Input: part model. Units: mm. Frame: model coordinates. A direction names the side the tool comes from. Coordinates: 2 decimals unless noted, no trailing zeros. Order: outer loops, then holes, each group sorted by start corner. A loop starts at its lowest first (then second) coordinate and runs counter-clockwise, first axis right, second up. Notation, with made-up numbers: (85.25, 70) -> (128.25, 70) arc R10 ccw to (128.25, 87) -> close; hole circle Ø4 at (25.5, 35). An arc over 180 degrees is marked (long way). Use one line per item in the form item = value. Start each with the question number.
1) Draft query along Y for faces 1 (the flat face through (-61.7, -38.656, 6.3)), 2 (the flat face through (-59.664, -5, 6)), 3 (the cylindrical face through (35.26, -34.87, 6.44)), 4 (the flat face through (-47, -1.432, 6)). Return one class per face: pulls with the +Y half, pulls with the -Y half, needs draft (parallel to the pull), parting line crosses it, or undercut.
2) Pin query (flat end, axial travel): pin 1 (3 mm diameter, centred on y = -6, z = 5, fed in from +X); pin 2 (7 mm diameter, centred on y = -5, z = 4, fed in from -X); pin 3 (4 mm diameter, centred on x = -7.5, z = 9, fed in from +Y). Return the tip coordinate at first contact, or that it passes through.
3) Section query A-A on y = -5.5. Output: boundary loops of the cut face in (x, z).
4) Section query D-D on x = -25.5. Output: boundary loops of the cut face in (y, z), then the cut area to 3 significant figures.
5) Section query B-B on z = 6.35. Count the separate pieces of the cut face and the enclosed holes in it, then the cut area to 3 significant figures.
6) Ray query, line 1 along Y through (x, z) = (-59, 1.5); line 2 along X through (y, z) = (-5.5, 6.35); line 3 along Z through (x, y) = (-52, -4). Return the intervals inside material, ascending.
7) Access query for faces 5 (the flat face through (47.2, -7.782, 7.7)), 6 (the flat face through (50.78, -5, 6)), 7 (the cylindrical face through (-48.168, -4.562, 5.129)). Directions: +Z, -Z, +X, -X, +Y, -Y. A direction counts if a zero-diameter tool reaches every point of the face in a straight line with its end or side. Return the directions, or none.
8) Section query C-C on x = 18. Output: boundary loops of the cut face in (y, z), then the cut area to 3 significant figures.
Autodesk Inventor part; units mm, degrees
ref_plane "YZ Plane" through (0, 0, 0) normal (1, 0, 0) x (0, 1, 0)
ref_plane "XZ Plane" through (0, 0, 0) normal (0, 1, 0) x (-1, 0, 0)
ref_plane "XY Plane" through (0, 0, 0) normal (0, 0, 1) x (1, 0, 0)
sketch "Sketch1" plane through (0, 0, 0) normal (0, 0, 1) x (1, 0, 0)
  arc A0 (-39.344, -1.4316) -> (30.4598, -1.4316) centre (-4.4421, -0.1616) ccw
  line L0 (-39.344, -1.4316) -> (-39.3671, -1.4316)
  line L1 (-39.344, -1.4316) -> (-52.044, -1.4316)
  line L2 (30.4598, -1.4316) -> (43.1598, -1.4316)
  arc A1 (-46.964, -22.4724) -> (38.0798, -22.4724) centre (-4.4421, -0.1616) ccw
  line L3 (-4.4421, -48.1813) -> (-4.4421, -51.3563)
  line L4 (-4.4421, -51.3563) -> (-72.364, -51.3563)
  line L5 (-4.4421, -51.3563) -> (63.4798, -51.3563)
  line L6 (-52.044, -1.4316) -> (-59.664, -1.4316)
  line L7 (43.1598, -1.4316) -> (50.7798, -1.4316)
  line L8 (30.4598, -1.4316) -> (38.0798, -1.4316)
  line L9 (38.0798, -1.4316) -> (38.0798, -22.4724)
  line L10 (-39.344, -1.4316) -> (-45.694, -1.4316)
  line L11 (-39.344, -1.4316) -> (-46.964, -1.4316)
  line L12 (-46.964, -1.4316) -> (-46.964, -22.4724)
  line L13 (-46.964, -7.7816) -> (-59.664, -7.7816)
  line L14 (-59.664, -7.7816) -> (-59.664, -1.4316)
  line L15 (38.0798, -7.7816) -> (50.7798, -7.7816)
  line L16 (50.7798, -7.7816) -> (50.7798, -1.4316)
  line L17 (-72.364, -51.3563) -> (-72.364, -38.6563)
  line L18 (63.4798, -51.3563) -> (63.4798, -38.6563)
  line L19 (-72.364, -38.6563) -> (-33.1483, -38.6563)
  line L20 (63.4798, -38.6563) -> (24.2642, -38.6563)
  point P0 (0, 0)
  dimension "d0" = 69.85
  dimension "d1" = 12.7
  dimension "d2" = 12.7
  dimension "d3" = 3.175
  dimension "d4" = 7.62
  dimension "d5" = 7.62
  dimension "d6" = 7.62
  dimension "d7" = 7.62
  dimension "d8" = 6.35
  dimension "d9" = 6.35
  dimension "d10" = 12.7
  dimension "d11" = 12.7
  dimension "d12" = 12.7
  dimension "d13" = 12.7
extrude "Extrusion1" add sketch "Sketch1" along normal blind 12.7
fillet "Fillet1" radius 7.62 2 edges at (24.2642, -38.6563, 6.35) (-33.1483, -38.6563, 6.35)
fillet "Fillet2" radius 25.4 2 edges at (-46.964, -22.4724, 6.35) (38.0798, -22.4724, 6.35)
sketch "Sketch2" plane through (-59.664, -1.4316, 0) normal (0, 1, 0) x (1, 0, 0)
  line L0 (20.32, 0) -> (20.32, -12.7)
  line L1 (0, 0) -> (20.32, 0)
  circle A0 centre (7.62, -6.35) radius 4.064
  circle A1 centre (102.8238, -6.35) radius 4.064
  line L2 (90.1238, 0) -> (90.1238, -12.7)
  line L3 (-12.7, 0) -> (-12.7, -12.7)
  line L4 (-12.7, -12.7) -> (0, -12.7)
  line L5 (0, -12.7) -> (0, 0)
  line L6 (0, 0) -> (-12.7, 0)
  line L7 (-12.7, 0) -> (-12.7, -12.7)
  line L8 (110.4438, 0) -> (110.4438, -12.7)
  line L9 (-12.7, 0) -> (123.1438, 0)
  line L10 (110.4438, -12.7) -> (123.1438, -12.7)
  line L11 (123.1438, -12.7) -> (123.1438, 0)
  line L12 (123.1438, 0) -> (110.4438, 0)
  line L13 (110.4438, 0) -> (110.4438, -12.7)
  circle A2 centre (-6.35, -6.35) radius 4.064
  circle A3 centre (116.7892, -6.35) radius 4.064
  point P0 (59.664, 0)
  dimension "d18" = 12.7
  dimension "d19" = 8.128
  dimension "d20" = 12.7
  dimension "d21" = 8.128
  dimension "d22" = 8.128
  dimension "d23" = 8.128
  dimension "d28" = 123.1392
extrude "Extrusion2" cut sketch "Sketch2" against normal blind 25.4 contours A0 | A1
extrude "Extrusion3" cut sketch "Sketch2" against normal blind 76.2 contours A2 | A3
properties part number "REAL MOTOR MOUNT 2.75 BOTTOM"
Answers below:
q1.face_1 = undercut
q1.face_2 = needs draft
q1.face_3 = undercut
q1.face_4 = pulls with the +Y half
q2.pin_1 = 50.78
q2.pin_2 = -59.66
q2.pin_3 = -34.72
q3.outline = (-59.66, 0) -> (-38.96, 0) -> (-38.96, 12.7) -> (-59.66, 12.7) -> close; (30.07, 0) -> (50.78, 0) -> (50.78, 12.7) -> (30.07, 12.7) -> close; hole circle Ø8.13 at (-52.04, 6.35); hole circle Ø8.13 at (43.16, 6.35)
q4.outline = (-51.36, 0) -> (-28.02, 0) -> (-28.02, 12.7) -> (-51.36, 12.7) -> close
q4.area = 296 mm^2
q5.separate_pieces = 5
q5.enclosed_holes = 0
q5.area = 2,830 mm^2
q6.line_1 = -51.36 to -38.66, -7.78 to -1.43
q6.line_2 = -59.66 to -56.11, -47.98 to -38.96, 30.07 to 39.1, 47.22 to 50.78
q6.line_3 = 0 to 2.29, 10.41 to 12.7
q7.face_5 = +Z, -Z, +X
q7.face_6 = +Z, -Z, +X, +Y
q7.face_7 = +Y
q8.outline = (-51.36, 0) -> (-26.92, 0) -> (-26.92, 12.7) -> (-51.36, 12.7) -> close
q8.area = 310 mm^2
